Check sheet for the modelled part. Datum: model origin and axes. Units: mm. Face numbers are marked on the shaded views. Round coordinates to 2 decimals unless told otherwise and drop trailing zeros. Order: outer loops, then holes, each group sorted by start corner. A loop starts at its lowest first (then second) coordinate and runs counter-clockwise, first axis right, second up. Notation, with made-up numbers: (-33.75, 2) -> (-1.75, 2) arc R19 cw to (-1.75, 13) -> close; hole circle Ø9 at (57.25, 71.25). An arc over 180 degrees is marked (long way). Answer as CSV lines item,"result". Start each with the question number.
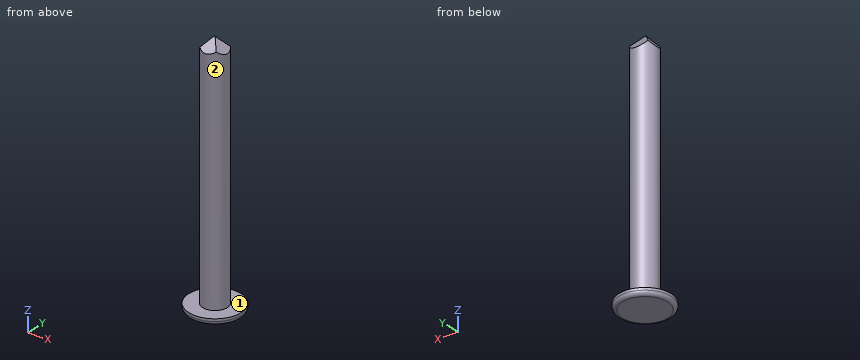
from build123d import *

# Parameters (mm, degrees)
F0_R          = 0.5
F1_DEPTH      = 10
F0_R_2        = 1.057388
F2_DEPTH      = 0.25
F3_R          = 0.15
F5_DEPTH      = 25
F5_DEPTH_BACK = 25
F7_DEPTH      = 25
F7_DEPTH_BACK = 25


with BuildPart() as f1:
    # F0 (on Top) → F1 (new body)
    with BuildSketch(Plane.XY):
        Circle(F0_R)
    extrude(amount=F1_DEPTH)

    # F0 (on Top) → F2 (join)
    with BuildSketch(Plane.XY):
        Circle(F0_R_2)
        Circle(F0_R, mode=Mode.SUBTRACT)
    extrude(amount=F2_DEPTH)

    # F3
    f3_edges = [f1.edges().sort_by_distance(p)[0] for p in [
        (-1.057388, 0, 0),
    ]]
    fillet(f3_edges, radius=F3_R)

    # F4 (on Right) → F5 (cut, two sides)
    with BuildSketch(Plane.YZ) as f5_sk:
        Polygon((-0.958076, 9.147321), (-0.022735, 9.998414), (0.690646, 9.140222), (0.690646, 10.352595), (-0.869291, 10.392135), align=None)
    extrude(amount=F5_DEPTH, mode=Mode.SUBTRACT)
    extrude(f5_sk.sketch, amount=-F5_DEPTH_BACK, mode=Mode.SUBTRACT)

    # F6 (on Front) → F7 (cut, two sides)
    with BuildSketch(Plane.XZ) as f7_sk:
        Polygon((-1.2872, 8.500885), (0, 10.019018), (1.330554, 8.673213), (1.125401, 10.741157), (-1.2872, 10.741157), align=None)
    extrude(amount=F7_DEPTH, mode=Mode.SUBTRACT)
    extrude(f7_sk.sketch, amount=-F7_DEPTH_BACK, mode=Mode.SUBTRACT)


solid = f1.part
1) Material ranges on line 1 along Z through (x, y) = (-0.5, -0.5); line 2 along X through (y, z) = (0, 1.5), recorded low to high.
2) Mould release check, pull along Y, two halves, no side actions. Record for the marked faces 1 and 2: released by +Y, released by -Y, zero draft, split by the parting line, or undercut.
3) Section check A-A on z = 7. Record the cut outline in (x, y), then the cut area to 3 significant figures.
Solutions:
1,line 1,"z = 0 to 0.25"
1,line 2,"x = -0.5 to 0.5"
2,face 1,"zero draft"
2,face 2,"split by the parting line"
3,outline,"circle Ø1 at (0, 0)"
3,area,"0.785 mm^2"
